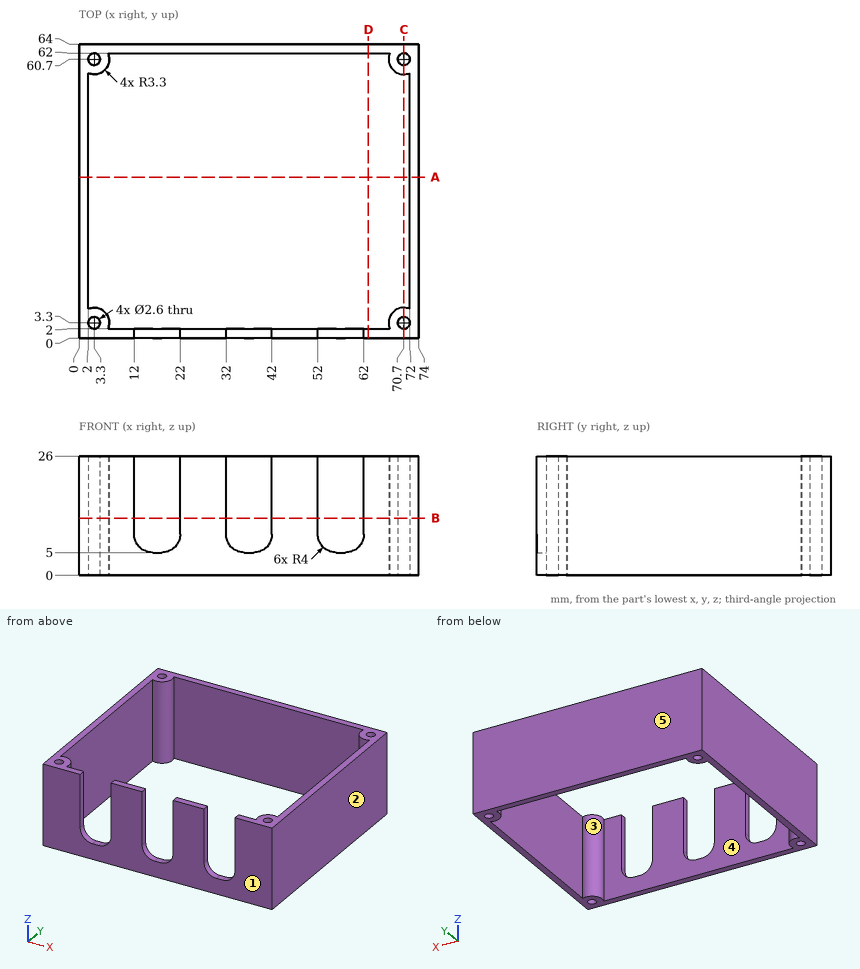
Job drawing, mm, ordinate dimensions from the low corner. One solid piece. A direction names the side the tool comes from. Round coordinates to 2 decimals unless told otherwise and drop trailing zeros. Write each loop counter-clockwise with the first axis right and the second up, starting at its lowest first coordinate (ties: lowest second). Pieces come first, ordered by that corner, then holes. Notation, with made-up numbers: (58.25, 63.5) -> (67.25, 63.5) arc R16 cw to (67.25, 93.5) -> close; hole circle Ø11 at (16, 2). An arc over 180 degrees is marked (long way). Answer as a JSON object with one key per item and string values.
(1) Which spindle directions (+Z, -Z, +X, -X, +Y, -Y) get a long thin tool onto all of the face, cutting with end or side? Do the marked faces 4 and 5. Say none if no direction does.
Reported:
{"face 4": "+Z, -Z", "face 5": "+Z, -Z, +X, -X, +Y"}
(2) Probe probe 1 along Y at (x, z) = (3.3, 12); probe 2 along X at (y, z) = (47, 15.5); probe 3 along X at (y, z) = (61, 18.5). List the from-to ranges inside material, lowest first. Write a range as [from, to].
Reported:
{"probe 1": "y = [0, 2], [4.6, 6.6], [57.4, 59.4], [62, 64]", "probe 2": "x = [0, 2], [72, 74]", "probe 3": "x = [0, 2.04], [4.56, 6.59], [67.41, 69.44], [71.96, 74]"}
(3) Band-saw the part on C-C, the plane x = 70.7. List the corners of the cut face in (y, z), then the cut area to 3 significant figures.
Reported:
{"outline": "(0, 0) -> (2, 0) -> (2, 26) -> (0, 26) -> close; (4.6, 0) -> (6.6, 0) -> (6.6, 26) -> (4.6, 26) -> close; (57.4, 0) -> (59.4, 0) -> (59.4, 26) -> (57.4, 26) -> close; (62, 0) -> (64, 0) -> (64, 26) -> (62, 26) -> close", "area": "208 mm^2"}
(4) Two-plate mould, pull along Y, no slides. Class the marked faces 1, 2 and 3: +Y half, -Y half, draft (parallel to the pull), parting line (faces both ways), or undercut.
Reported:
{"face 1": "-Y half", "face 2": "draft", "face 3": "undercut"}
(5) Band-saw the part on B-B, the plane z = 12.5. List the corners of the cut face in (x, y).
Reported:
{"outline": "(0, 0) -> (12, 0) -> (12, 2) -> (6.33, 2) arc R3.3 ccw to (2, 6.33) -> (2, 57.67) arc R3.3 ccw to (6.33, 62) -> (67.67, 62) arc R3.3 ccw to (72, 57.67) -> (72, 6.33) arc R3.3 ccw to (67.67, 2) -> (62, 2) -> (62, 0) -> (74, 0) -> (74, 64) -> (0, 64) -> close; (22, 0) -> (32, 0) -> (32, 2) -> (22, 2) -> close; (42, 0) -> (52, 0) -> (52, 2) -> (42, 2) -> close; hole circle Ø2.6 at (3.3, 3.3); hole circle Ø2.6 at (3.3, 60.7); hole circle Ø2.6 at (70.7, 3.3); hole circle Ø2.6 at (70.7, 60.7)"}
(6) Band-saw the part on A-A, the plane y = 35. List the corners of the cut face in (x, z), then the cut area to 3 significant figures.
Reported:
{"outline": "(0, 0) -> (2, 0) -> (2, 26) -> (0, 26) -> close; (72, 0) -> (74, 0) -> (74, 26) -> (72, 26) -> close", "area": "104 mm^2"}
(7) Band-saw the part on D-D, the plane x = 63. List the corners of the cut face in (y, z), then the cut area to 3 significant figures.
Reported:
{"outline": "(0, 0) -> (2, 0) -> (2, 26) -> (0, 26) -> close; (62, 0) -> (64, 0) -> (64, 26) -> (62, 26) -> close", "area": "104 mm^2"}
(8) Pin check, flat tips, straight feed: P1, Ø0.6, axis at x = 57, y = 0.5, coming from the +Z side; P2, Ø1.5, axis at x = 20.5, z = 18, coming from the -Y side; P3, Ø2, axis at x = 3.3, y = 3.3, coming from the +Z side. Stop position of each tip, or through.
Reported:
{"P1": "stops at z = 5", "P2": "stops at y = 62", "P3": "passes through"}
